from build123d import *

# Parameters (mm, degrees)
FILLET2_R = 0.4


with BuildPart() as part:
    # Sketch1 → Base (revolve)
    with BuildSketch(Plane(origin=(0, 0, 0), x_dir=(1, 0, 0), z_dir=(0, 1, 0)), mode=Mode.PRIVATE) as base_sk:
        Polygon((2.2, 2), (12, 2), (12, 0), (0, 0), (0, 4), (0.2, 4), align=None)
    revolve(base_sk.sketch.rotate(Axis((-6.506452013, 0, 0), (1, 0, 0)), 180), axis=Axis((-6.506452013, 0, 0), (1, 0, 0)))

    # Sketch3 → Cut-Revolve1 (revolve, cut)
    with BuildSketch(Plane.XY, mode=Mode.PRIVATE) as cut_revolve1_sk:
        Polygon((12.15755877, 0), (12.15755877, 20), (-8, 20), (12, 0), align=None)
    revolve(cut_revolve1_sk.sketch.rotate(Axis((4.883468835, 0, 0), (1, 0, 0)), 90), axis=Axis((4.883468835, 0, 0), (1, 0, 0)), mode=Mode.SUBTRACT)

    # Fillet2
    fillet2_edges = [part.edges().sort_by_distance(p)[0] for p in [
        (2.2, 0, -2),
    ]]
    fillet(fillet2_edges, radius=FILLET2_R)

    # Sketch2 → Cut-Loft1 section 0
    with BuildSketch(Plane(origin=(0, -0.680816871, 0.306758275), x_dir=(0, 0, 1), z_dir=(-1, 0, 0)), mode=Mode.PRIVATE) as cut_loft1_s0:
        with BuildLine():
            Line((-0.786758275, 1.160816871), (-2.706758275, 1.160816871))
            Line((-2.706758275, 1.160816871), (-2.706758275, 0.200816871))
            Line((-2.706758275, 0.200816871), (-0.786758275, 0.200816871))
            Line((-0.786758275, 0.200816871), (-0.786758275, -1.719183129))
            Line((-0.786758275, -1.719183129), (0.173241725, -1.719183129))
            Line((0.173241725, -1.719183129), (0.173241725, 0.200816871))
            Line((0.173241725, 0.200816871), (2.093241725, 0.200816871))
            Line((2.093241725, 0.200816871), (2.093241725, 1.160816871))
            Line((2.093241725, 1.160816871), (0.173241725, 1.160816871))
            Line((0.173241725, 1.160816871), (0.173241725, 3.080816871))
            Line((0.173241725, 3.080816871), (-0.786758275, 3.080816871))
            Line((-0.786758275, 3.080816871), (-0.786758275, 1.160816871))
        make_face()
    loft([cut_loft1_s0.sketch, Vertex(2.45, 0, 0)], mode=Mode.SUBTRACT)


solid = part.part
Design review of the part built by this model. Coordinates are the model's own, in mm. A direction names the side the tool comes from. Give positions to 0.01 mm unless a question says otherwise; leave off trailing zeros. Order: outer loops, then holes, each group sorted by start corner. A loop starts at its lowest first (then second) coordinate and runs counter-clockwise, first axis right, second up. Notation, with made-up numbers: (35.25, 63.5) - (87.25, 63.5) arc R14 cw to (87.25, 89.5) - close; hole circle Ø2 at (-4.75, 74). An arc over 180 degrees is marked (long way). Use CSV: the item, a comma, the result in double quotes. Start each with the question number.
Q1. Machinability: for faces 5 (the face through (6.236, 0.766, 1.847)), 6 (the face through (0.777, 0.939, -0.328)), which of the approach directions +Z, -Z, +X, -X, +Y, -Y give a long, thin tool a straight path to every point of the face, cutting with its end or side? Answer none if there is none.
Q2. For P1, Ø1, axis at x = 7.5, y = 3, coming from the -Z side; P2, Ø3, axis at x = 2, y = -1, coming from the +Z side; P3, Ø2, axis at x = 9.5, z = -1, coming from the -Y side; P4, Ø1.5, axis at x = 3.5, y = -2, coming from the +Z side, all flat-tipped, find the tip position at first contact; note any pin that passes through.
Q3. Draft analysis for pull direction Z (two halves, no side actions). For faces 1 (the face through (0.777, -0.328, -0.939)), 2 (the face through (0, 1, -1)), 3 (the face through (0.777, -0.328, 0.928)), 4 (the face through (11.5, 0.3, -0.4)), state which applies: pulls with the +Z half, pulls with the -Z half, needs draft (parallel to the pull), parting line crosses it, or undercut.
Q4. Take a section at B-B (x = 7). State the section outline as (y, z) points.
Q5. Take a section at A-A (x = 1). State the section outline as (y, z) points, and give its area (3 significant figures).
Q6. For line 1 (X direction, y = -3.5, z = 1.25); line 2 (Z direction, x = 0.5, y = -1.5); line 3 (Z direction, x = 7, y = -0.25), list the stretches that pass through material, from the lowest coordinate up.
Calculated:
1,face 5,"+X"
1,face 6,"-X"
2,P1,"passes through"
2,P2,"stops at z = 3.6"
2,P3,"stops at y = -2"
2,P4,"stops at z = 1.56"
3,face 1,"undercut"
3,face 2,"needs draft"
3,face 3,"undercut"
3,face 4,"parting line crosses it"
4,outline,"circle Ø4 at (0, 0)"
5,outline,"circle Ø6.4 at (0, 0); hole (-1.42, -0.28) - (-0.28, -0.28) - (-0.28, -1.42) - (0.28, -1.42) - (0.28, -0.28) - (1.42, -0.28) - (1.42, 0.28) - (0.28, 0.28) - (0.28, 1.42) - (-0.28, 1.42) - (-0.28, 0.28) - (-1.42, 0.28) - close"
5,area,"29.3 mm²"
6,line 1,"x = 0 to 0.48"
6,line 2,"z = -3.38 to -0.38, 0.38 to 3.38"
6,line 3,"z = -1.98 to 1.98"
